Autodesk Inventor part; units mm, degrees
ref_plane "YZ Plane" through (0, 0, 0) normal (1, 0, 0) x (0, 1, 0)
ref_plane "XZ Plane" through (0, 0, 0) normal (0, 1, 0) x (-1, 0, 0)
ref_plane "XY Plane" through (0, 0, 0) normal (0, 0, 1) x (1, 0, 0)
sketch "Esboço2" plane through (0, 0, 0) normal (0, 0, 1) x (1, 0, 0)
  line L0 (-15, 10) -> (15, 10)
  line L1 (15, 10) -> (15, -20)
  line L2 (15, -20) -> (-15, -20)
  line L3 (-15, -20) -> (-15, 10)
  line L4 (-15, 10) -> (15, -20) construction
  line L5 (15, 10) -> (-15, -20) construction
  point P0 (0, -5)
  dimension "d10" = 30
  dimension "d11" = 30
extrude "Extrusão1" add sketch "Esboço2" along normal blind 45
sketch "Esboço3" plane through (0, 0, 45) normal (0, 0, 1) x (1, 0, 0)
  line L0 (15, 10) -> (-15, 10)
  line L1 (0, 10) -> (0, -3.62)
  circle A0 centre (0, -3.62) radius 10.5
  point P0 (0, 0)
  dimension "d14" = 13.62
  dimension "d15" = 21
hole "Furo1" at (0, -3.62, 45) direction (0, 0, -1) diameter 12.5 end through all counterbore diameter 21.05 counterbore depth 32
sketch "Esboço4" plane through (-15, -20, 0) normal (0, -1, 0) x (1, 0, 0)
  line L0 (15, 0) -> (15, 45)
  line L1 (30, 45) -> (0, 45)
  circle A0 centre (15, 10) radius 1.6056 construction
  circle A1 centre (15, 35) radius 1.4692 construction
  line L2 (0, 0) -> (0, 45) construction
  line L3 (0, 22.5) -> (30, 22.5) construction
  line L4 (30, 0) -> (30, 45) construction
  dimension "d23" = 12.5
  dimension "d24" = 12.5
hole "Furo2" at (0, -20, 10) at (0, -20, 35) direction (0, 1, 0) diameter 3.242 depth 6 tip angle 118
properties part number "blocoSuporteRolamentosTeste"
The listing builds one solid part. Answer for the finished solid, in the listing's coordinates (mm). A direction names the side the tool comes from. Give positions to 0.01 mm unless a question says otherwise; leave off trailing zeros. Order: outer loops, then holes, each group sorted by start corner. A loop starts at its lowest first (then second) coordinate and runs counter-clockwise, first axis right, second up. Notation, with made-up numbers: (-15, 25.5) -> (31, 25.5) arc R21 ccw to (31, 62.5) -> close; hole circle Ø11 at (17.5, -17). An arc over 180 degrees is marked (long way). One line per item, written item: value.
1) Determine the mould class of faces 1 (the cylindrical face through (0.986, -16.968, 36.286)), 2 (the flat face through (0, -11, 0)), 3 (the flat face through (-15, -5, 22)) for opening direction X: pulls with the +X half, pulls with the -X half, needs draft (parallel to the pull), parting line crosses it, or undercut.
Reported:
face 1: undercut
face 2: needs draft
face 3: pulls with the -X half
2) Find the intervals of material crossed by line 1 (Z direction, x = 0, y = -16.6); line 2 (Y direction, x = 0, z = 30) (3 decimals); line 3 (Y direction, x = 0, z = 5.75), in increasing order.
Reported:
line 1: z = 0 to 8.38, 11.62 to 33.38, 36.62 to 45
line 2: y = -20 to -14.145, 6.905 to 10
line 3: y = -20 to -9.87, 2.63 to 10
3) Find section C-C, the plane x = 4. Determine the outline of the cut face in (y, z), plus the area to 3 significant figures.
Reported:
outline: (-20, 0) -> (-8.42, 0) -> (-8.42, 13) -> (-13.36, 13) -> (-13.36, 45) -> (-20, 45) -> close; (1.18, 0) -> (10, 0) -> (10, 45) -> (6.12, 45) -> (6.12, 13) -> (1.18, 13) -> close
area: 602 mm^2
4) Find section A-A, the plane y = -3.62. Determine the outline of the cut face in (x, z) (3 decimals).
Reported:
outline: (-15, 0) -> (-6.25, 0) -> (-6.25, 13) -> (-10.525, 13) -> (-10.525, 45) -> (-15, 45) -> close; (6.25, 0) -> (15, 0) -> (15, 45) -> (10.525, 45) -> (10.525, 13) -> (6.25, 13) -> close
5) A tool of negligible diameter and unlimited length cuts with its end or side. For faces 4 (the cylindrical face through (-3.16, -13.66, 28.78)), 5 (the flat face through (15, -5, 22)), 6 (the cylindrical face through (-0.07, -16.96, 11.62)), from which of +Z, -Z, +X, -X, +Y, -Y can it reach the whole face along a straight path? Write none if from no direction.
Reported:
face 4: +Z
face 5: +Z, -Z, +X, +Y, -Y
face 6: -Y
6) Find section D-D, the plane y = 6. Determine the outline of the cut face in (x, z).
Reported:
outline: (-15, 0) -> (15, 0) -> (15, 45) -> (4.27, 45) -> (4.27, 13) -> (-4.27, 13) -> (-4.27, 45) -> (-15, 45) -> close
7) Find section B-B, the plane z = 31. Determine the outline of the cut face in (x, y) (3 decimals).
Reported:
outline: (-15, -20) -> (15, -20) -> (15, 10) -> (-15, 10) -> close; hole circle Ø21.05 at (0, -3.62)
